from build123d import *

# Parameters (mm, degrees)
SKETCH_1_W               = 2
SKETCH_1_H               = 22
CUT_EXTRUDE_1_DEPTH      = 27.944387171
CUT_EXTRUDE_1_DEPTH_BACK = 27.944387171
SKETCH_2_W               = 17
SKETCH_2_H               = 4


with BuildPart() as part:
    # 草图1 → 旋转1 (revolve)
    with BuildSketch(Plane.XY, mode=Mode.PRIVATE) as revolve_1_sk:
        with Locations((10, 11)):
            Rectangle(SKETCH_1_W, SKETCH_1_H)
    revolve(revolve_1_sk.sketch.rotate(Axis((0, 25.51049322, 0), (0, -1, 0)), 90), axis=Axis((0, 25.51049322, 0), (0, -1, 0)))

    # 草图2 → 切除-拉伸1 (cut, two sides: drawn at the far end of the back side and taken through both)
    with BuildSketch(Plane.XY.offset(-CUT_EXTRUDE_1_DEPTH_BACK)):
        with Locations((3.12, 11)):
            Rectangle(SKETCH_2_W, SKETCH_2_H)
    extrude(amount=CUT_EXTRUDE_1_DEPTH + CUT_EXTRUDE_1_DEPTH_BACK, mode=Mode.SUBTRACT)


solid = part.part
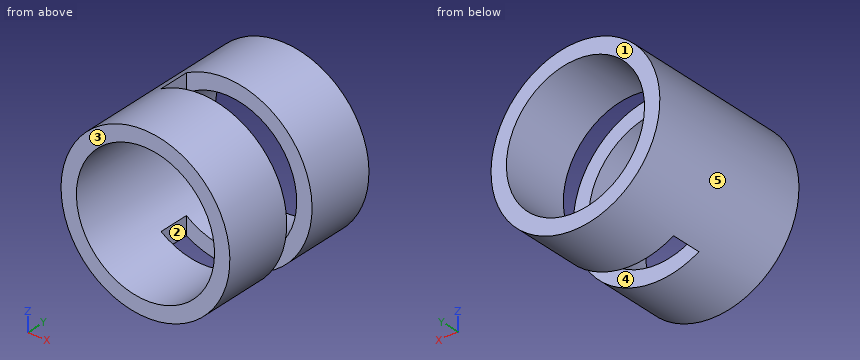
Geometry: final body of the model. Coordinates: model frame, mm. Face numbers are marked on the shaded views. A direction names the side the tool comes from. Give positions to 0.01 mm unless a question says otherwise; leave off trailing zeros. Loops run counter-clockwise (first coordinate to the right, second up) from the corner with the lowest first, then second, coordinate; pieces in that order, holes last. Notation, with made-up numbers: M -13,30 L 30,30 A27 ccw 30,53 Z; hole C -29.75,27.5 d8. An arc over 180 degrees is marked long. Put each result on its own line as item: value. Start each with the question number.
1) Access query for the marked faces 4 and 5. Directions: +Z, -Z, +X, -X, +Y, -Y. A direction counts if a zero-diameter tool reaches every point of the face in a straight line with its end or side. Return the directions, or none.
2) Cut plane C-C (y = 2). Output: boundary loops of the cut face in (x, z), then the cut area to 3 significant figures.
3) Cut plane A-A (x = 0). Output: boundary loops of the cut face in (y, z).
4) Contact query for flat-ended pins moving along their axis: pin 1 (1.9 mm diameter, centred on y = 11, z = -8.5, fed in from +X); pin 2 (1 mm diameter, centred on y = 10, z = -3, fed in from +X); pin 3 (1 mm diameter, centred on x = 4.5, z = 5, fed in from +Y); pin 4 (10 mm diameter, centred on x = -8, y = 8, fed in from +Z). Output: stop coordinate, or through.
5) Pull-direction query (Y, two-part tool) for the marked faces 1, 2 and 3; classes: pulls with the +Y half, pulls with the -Y half, needs draft (parallel to the pull), parting line crosses it, or undercut.
6) Cut plane D-D (z = 7.75). Output: boundary loops of the cut face in (x, y).
7) Ray query, line 1 along X through (y, z) = (13.75, 0); line 2 along Y through (x, z) = (-3.25, -10); line 3 along X through (y, z) = (20.5, 2.75). Return the intervals inside material, ascending.
8) Cut plane B-B (z = 0). Output: boundary loops of the cut face in (x, y), then the cut area to 3 significant figures.
Verdict:
1. face 4: +Z, -Z, +X
1. face 5: +Y, -Y
2. outline: C 0,0 d22; hole C 0,0 d18
2. area: 126 mm2
3. outline: M 0,-11 L 9,-11 L 9,-9 L 0,-9 Z; M 0,9 L 9,9 L 9,11 L 0,11 Z; M 13,-11 L 22,-11 L 22,-9 L 13,-9 Z; M 13,9 L 22,9 L 22,11 L 13,11 Z
4. pin 1: x = -5.38
4. pin 2: x = -8.29
4. pin 3: through
4. pin 4: z = 10.58
5. face 1: pulls with the +Y half
5. face 2: undercut
5. face 3: pulls with the -Y half
6. outline: M -7.81,0 L -4.58,0 L -4.58,9 L -5.38,9 L -5.38,13 L -4.58,13 L -4.58,22 L -7.81,22 Z; M 4.58,0 L 7.81,0 L 7.81,9 L 4.58,9 Z; M 4.58,13 L 7.81,13 L 7.81,22 L 4.58,22 Z
7. line 1: -11 to -9, 9 to 11
7. line 2: 0 to 9, 13 to 22
7. line 3: -10.65 to -8.57, 8.57 to 10.65
8. outline: M -11,0 L -9,0 L -9,22 L -11,22 Z; M 9,0 L 11,0 L 11,9 L 9,9 Z; M 9,13 L 11,13 L 11,22 L 9,22 Z
8. area: 80.0 mm2
